Input: part model. Units: mm. Frame: model coordinates. A direction names the side the tool comes from. Coordinates: 2 decimals unless noted, no trailing zeros. Loops run counter-clockwise (first coordinate to the right, second up) from the corner with the lowest first, then second, coordinate; pieces in that order, holes last. Notation, with made-up numbers: (-13, -22) -> (42, -22) arc R27 ccw to (42, -5) -> close; hole circle Ø9 at (75, -20). An arc over 180 degrees is marked (long way). Answer as a JSON object with one key per item and string values.
from build123d import *

# Parameters (mm, degrees)
BOSS_EXTRUDE1_DEPTH = 3
SKETCH3_R           = 1.6
SKETCH3_W           = 20
SKETCH3_H           = 3
SKETCH3_W_2         = 3
SKETCH3_H_2         = 10
ARDUINO_DEPTH       = 4
SKETCH6_R           = 1.6
CUT_EXTRUDE4_DEPTH  = 4
SKETCH8_R           = 1.6
CUT_EXTRUDE5_DEPTH  = 10
SKETCH9_R           = 1.6
SKETCH9_R_2         = 2.5
SKETCH9_W           = 3
SKETCH9_H           = 10
L298N_DEPTH         = 10
SKETCH11_W          = 150
SKETCH11_H          = 5
BOSS_EXTRUDE3_DEPTH = 60
FILLET1_R           = 10
SKETCH12_R          = 1.6
CUT_EXTRUDE6_DEPTH  = 10


with BuildPart() as part:
    # Sketch1 → Boss-Extrude1 (new body)
    with BuildSketch(Plane(origin=(0, 0, 0), x_dir=(1, 0, 0), z_dir=(0, 1, 0))):
        with BuildLine():
            Line((100, -40), (100, 10))
            Line((100, 10), (30, 170))
            Line((30, 170), (-30, 170))
            Line((-30, 170), (-100, 10))
            Line((-100, 10), (-100, -40))
            ThreePointArc((-100, -40), (-97.071067812, -47.071067812), (-90, -50))
            Line((-90, -50), (-75, -50))
            Line((-75, -50), (-75, -70))
            Line((-75, -70), (75, -70))
            Line((75, -70), (75, -50))
            Line((75, -50), (90, -50))
            ThreePointArc((90, -50), (97.071067812, -47.071067812), (100, -40))
        make_face()
    extrude(amount=BOSS_EXTRUDE1_DEPTH)

    # Sketch3 → arduino (cut, through all)
    with BuildSketch(Plane(origin=(0, 3, 0), x_dir=(1, 0, 0), z_dir=(0, 1, 0))):
        with Locations((-70.120983048, 12.737637313)):
            Circle(SKETCH3_R)
        with Locations((-71.220983048, -35.062362687)):
            Circle(SKETCH3_R)
        with Locations((-19.320983048, -2.462362687)):
            Circle(SKETCH3_R)
        with Locations((-19.320983048, -30.362362687)):
            Circle(SKETCH3_R)
        with Locations((-39.320983048, -41.562362687)):
            Rectangle(SKETCH3_W, SKETCH3_H)
        with Locations((-39.320983048, 19.237637313)):
            Rectangle(SKETCH3_W, SKETCH3_H)
        with Locations((-12.820983048, -25.362362687)):
            Rectangle(SKETCH3_W_2, SKETCH3_H_2)
    extrude(amount=-ARDUINO_DEPTH, mode=Mode.SUBTRACT)

    # Sketch6 → Cut-Extrude4 (cut, through all)
    with BuildSketch(Plane(origin=(0, 3, 0), x_dir=(1, 0, 0), z_dir=(0, 1, 0))):
        with Locations((12, 155)):
            Circle(SKETCH6_R)
        with Locations((-12, 155)):
            Circle(SKETCH6_R)
        with Locations((12, 125)):
            Circle(SKETCH6_R)
        with Locations((-12, 125)):
            Circle(SKETCH6_R)
    extrude(amount=-CUT_EXTRUDE4_DEPTH, mode=Mode.SUBTRACT)

    # Sketch8 → Cut-Extrude5 (cut)
    with BuildSketch(Plane(origin=(0, 3, 0), x_dir=(1, 0, 0), z_dir=(0, 1, 0))):
        with Locations((8, 10)):
            Circle(SKETCH8_R)
        with Locations((-8, 10)):
            Circle(SKETCH8_R)
        with Locations((-65, -60)):
            Circle(SKETCH8_R)
        with Locations((65, -60)):
            Circle(SKETCH8_R)
    extrude(amount=-CUT_EXTRUDE5_DEPTH, mode=Mode.SUBTRACT)

    # Sketch9 → l298n (cut)
    with BuildSketch(Plane(origin=(0, 3, 0), x_dir=(1, 0, 0), z_dir=(0, 1, 0))):
        with Locations((20, 72)):
            Circle(SKETCH9_R)
        with Locations((-20, 72)):
            Circle(SKETCH9_R)
        with Locations((45, 10)):
            Circle(SKETCH9_R)
        with Locations((81.998174007, 10.367586933)):
            Circle(SKETCH9_R)
        with Locations((82.36576094, -26.630587074)):
            Circle(SKETCH9_R)
        with Locations((45.367586933, -26.998174007)):
            Circle(SKETCH9_R)
        with Locations((-68.125, 50)):
            Circle(SKETCH9_R)
        with Locations((68.125, 50)):
            Circle(SKETCH9_R)
        with Locations((55, 25)):
            Circle(SKETCH9_R_2)
        with Locations((55.367586933, -41.998174007)):
            Circle(SKETCH9_R_2)
        with Locations((0, 27)):
            Circle(SKETCH9_R_2)
        with Locations((30, 0)):
            Rectangle(SKETCH9_W, SKETCH9_H)
    extrude(amount=-L298N_DEPTH, mode=Mode.SUBTRACT)

    # Sketch11 → Boss-Extrude3 (add)
    with BuildSketch(Plane(origin=(0, 43, 0), x_dir=(1, 0, 0), z_dir=(0, 1, 0))):
        with Locations((0, -72.5)):
            Rectangle(SKETCH11_W, SKETCH11_H)
    extrude(amount=-BOSS_EXTRUDE3_DEPTH)

    # Fillet1
    fillet1_edges = [part.edges().sort_by_distance(p)[0] for p in [
        (-75, -17, 72.5),
        (75, -17, 72.5),
        (-75, 43, 72.5),
        (75, 43, 72.5),
    ]]
    fillet(fillet1_edges, radius=FILLET1_R)

    # Sketch12 → Cut-Extrude6 (cut)
    with BuildSketch(Plane.XY.offset(75)):
        with Locations((-65, -10)):
            Circle(SKETCH12_R)
        with Locations((-51, -10)):
            Circle(SKETCH12_R)
        with Locations((-65, -4)):
            Circle(SKETCH12_R)
        with Locations((-65, 6)):
            Circle(SKETCH12_R)
        with Locations((-65, 12)):
            Circle(SKETCH12_R)
        with Locations((-51, 12)):
            Circle(SKETCH12_R)
        with Locations((-51, 6)):
            Circle(SKETCH12_R)
        with Locations((-51, -4)):
            Circle(SKETCH12_R)
        with Locations((51, -10)):
            Circle(SKETCH12_R)
        with Locations((65, -10)):
            Circle(SKETCH12_R)
        with Locations((51, -4)):
            Circle(SKETCH12_R)
        with Locations((51, 6)):
            Circle(SKETCH12_R)
        with Locations((51, 12)):
            Circle(SKETCH12_R)
        with Locations((65, -4)):
            Circle(SKETCH12_R)
        with Locations((65, 6)):
            Circle(SKETCH12_R)
        with Locations((65, 12)):
            Circle(SKETCH12_R)
        with Locations((-8, 25)):
            Circle(SKETCH12_R)
        with Locations((8, 25)):
            Circle(SKETCH12_R)
    extrude(amount=-CUT_EXTRUDE6_DEPTH, mode=Mode.SUBTRACT)


solid = part.part
1. Pin query (flat end, axial travel): P1, Ø0.9, axis at x = 30.5, y = 1, coming from the -Z side; P2, Ø4, axis at x = -17, z = -75.5, coming from the -Y side; P3, Ø4, axis at x = 24, y = 30, coming from the -Z side; P4, Ø2.5, axis at x = 51, y = 12, coming from the -Z side. Return the tip coordinate at first contact, or that it passes through.
Reply:
{"P1": "stops at z = -169.89", "P2": "stops at y = 0", "P3": "stops at z = 70", "P4": "passes through"}
2. Mould query, pull axis Z, two halves, no side actions, for faces 1 (the face through (56.34, 1.52, -27.11)), 2 (the face through (71.99, -14.15, 72.46)), 3 (the face through (-1, 13, 75)). Classes: pulls with the +Z half, pulls with the -Z half, needs draft (parallel to the pull), parting line crosses it, or undercut.
Reply:
{"face 1": "undercut", "face 2": "needs draft", "face 3": "pulls with the +Z half"}
3. Access query for faces 4 (the face through (-75, 12, 71)), 5 (the face through (-1, 0, -52)), 6 (the face through (-1, 23, 70)), 7 (the face through (-1, -17, 72)), 8 (the face through (75, 12, 71)). Directions: +Z, -Z, +X, -X, +Y, -Y. A direction counts if a zero-diameter tool reaches every point of the face in a straight line with its end or side. Return the directions, or none.
Reply:
{"face 4": "+Z, -X, +Y, -Y", "face 5": "-Z, +X, -X, -Y", "face 6": "-Z, +X, -X, +Y", "face 7": "+Z, -Z, +X, -X, -Y", "face 8": "+Z, +X, +Y, -Y"}
4. Section query A-A (x = -55.5). Return loops of the section in (y, z), plus the area to 3 significant figures.
Reply:
{"outline": "(-17, 70) -> (0, 70) -> (0, -111.71) -> (3, -111.71) -> (3, 70) -> (43, 70) -> (43, 75) -> (-17, 75) -> close", "area": "845 mm2"}
5. Section query B-B (z = -141). Return loops of the section in (x, y), plus the area to 3 significant figures.
Reply:
{"outline": "(-42.69, 0) -> (42.69, 0) -> (42.69, 3) -> (-42.69, 3) -> close", "area": "256 mm2"}
6. Line query: line 1 along Z through (x, y) = (-22, -4); line 2 along Y through (x, z) = (57, 30.5). Output: solid intervals per line, ascending.
Reply:
{"line 1": "z = 70 to 75", "line 2": "y = 0 to 3"}
